Could you check a few things on this model? Use its own coordinates, in mm. A direction names the side the tool comes from. Give positions to 0.01 mm unless a question says otherwise; leave off trailing zeros. Write each loop counter-clockwise with the first axis right and the second up, starting at its lowest first coordinate (ties: lowest second). Pieces come first, ordered by that corner, then holes. Notation, with made-up numbers: M 44,51.25 L 99,51.25 A16 ccw 99,66.25 Z; hole C 47,34.25 d2. An arc over 180 degrees is marked long. Answer as CSV lines item,"result". Start each with the question number.
from build123d import *

# Parameters (mm, degrees)
F0_W     = 131.2458962202
F0_H     = 85.1092487574
F1_DEPTH = 38.1
F2_W     = 122.6490065455
F2_H     = 66.7691901326
F3_DEPTH = 109.982
F4_R     = 8.1771007469
F5_DEPTH = 175.514
F6_W     = 64.7632628679
F6_H     = 36.3935176283
F7_DEPTH = 112.776


with BuildPart() as f1:
    # F0 (on Front) → F1 (new body, symmetric)
    with BuildSketch(Plane.XZ):
        Rectangle(F0_W, F0_H)
    extrude(amount=F1_DEPTH, both=True)

    # F2 (on face) → F3 (cut)
    with BuildSketch(Plane.XY.offset(42.5546243787)):
        Rectangle(F2_W, F2_H)
    extrude(amount=-F3_DEPTH, mode=Mode.SUBTRACT)

    # F4 (on face) → F5 (cut)
    with BuildSketch(Plane.YZ.offset(65.6229481101)):
        Circle(F4_R)
    extrude(amount=-F5_DEPTH, mode=Mode.SUBTRACT)

    # F6 (on face) → F7 (cut)
    with BuildSketch(Plane.XZ.offset(38.1)):
        with Locations((5.444701761, 30.6622525677)):
            Rectangle(F6_W, F6_H)
    extrude(amount=-F7_DEPTH, mode=Mode.SUBTRACT)


solid = f1.part
1. Imagine slicing it at B-B, the plane x = 55.5. Please give me the cut outline in (y, z).
2. Thinking about a two-plate mould opening in X: for faces 1 (the flat face through (-1, 33.385, -9)), 2 (the flat face through (65.623, -9, -1)), 3 (the flat face through (-62, 0, 42.555)), 4 (the flat face through (5, 36, 12.465)), which applies, pulls with the +X half, pulls with the -X half, needs draft (parallel to the pull), parting line crosses it, or undercut?
3. Please list where these lines run through material, in increasing order: line 1 (Y direction, x = -57.5, z = 27); line 2 (X direction, y = 7.5, z = -11.5); line 3 (Z direction, x = 62.6, y = 0).
4. Imagine slicing it at D-D, the plane y = -21. Please give me the cut outline in (x, z).
5. Will these pins go through, and if not, where does the flat tip stop? P1, Ø2.5, axis at x = 16.5, y = 36, coming from the +Z side; P2, Ø10, axis at y = 0, z = 0, coming from the +X side.
6. Imagine slicing it at C-C, the plane z = 25. Please give me the cut outline in (x, y), plus the area to 3 significant figures.
7. Imagine slicing it at A-A, the plane y = 0. Please give me the cut outline in (x, z).
8. On a 3-axis mill with a long thin cutter (end or side, diameter ignored), from which of +Z, -Z, +X, -X, +Y, -Y can I reach the whole of each face in a straight line? I mean faces 5 (the flat face through (5, -36, 12.465)), 6 (the cylindrical face through (63.5, 7.8, 2.46)), 7 (the flat face through (61.325, 0, 10)). Say none if no direction works.
Solutions:
1,outline,"M -38.1,-42.55 L -33.38,-42.55 L -33.38,42.55 L -38.1,42.55 Z; M 33.38,-42.55 L 38.1,-42.55 L 38.1,42.55 L 33.38,42.55 Z"
2,face 1,"undercut"
2,face 2,"pulls with the +X half"
2,face 3,"needs draft"
2,face 4,"undercut"
3,line 1,"-38.1 to -33.38, 33.38 to 38.1"
3,line 2,"-65.62 to -61.32, 61.32 to 65.62"
3,line 3,"-42.55 to -8.18, 8.18 to 42.55"
4,outline,"M -65.62,-42.55 L -61.32,-42.55 L -61.32,42.55 L -65.62,42.55 Z; M 61.32,-42.55 L 65.62,-42.55 L 65.62,42.55 L 61.32,42.55 Z"
5,P1,"z = 12.47"
5,P2,"through"
6,outline,"M -65.62,-38.1 L -26.94,-38.1 L -26.94,-33.38 L -61.32,-33.38 L -61.32,33.38 L -26.94,33.38 L -26.94,38.1 L -65.62,38.1 Z; M 37.83,-38.1 L 65.62,-38.1 L 65.62,38.1 L 37.83,38.1 L 37.83,33.38 L 61.32,33.38 L 61.32,-33.38 L 37.83,-33.38 Z"
6,area,"1,200 mm²"
7,outline,"M -65.62,-42.55 L -61.32,-42.55 L -61.32,-8.18 L -65.62,-8.18 Z; M -65.62,8.18 L -61.32,8.18 L -61.32,42.55 L -65.62,42.55 Z; M 61.32,-42.55 L 65.62,-42.55 L 65.62,-8.18 L 61.32,-8.18 Z; M 61.32,8.18 L 65.62,8.18 L 65.62,42.55 L 61.32,42.55 Z"
8,face 5,"+Z, +Y, -Y"
8,face 6,"+X, -X"
8,face 7,"+Z, -Z"
